Autodesk Inventor part; units mm, degrees
ref_plane "YZ Plane" through (0, 0, 0) normal (1, 0, 0) x (0, 1, 0)
ref_plane "XZ Plane" through (0, 0, 0) normal (0, 1, 0) x (-1, 0, 0)
ref_plane "XY Plane" through (0, 0, 0) normal (0, 0, 1) x (1, 0, 0)
sketch "Sketch1" plane through (0, 0, 0) normal (0, 0, 1) x (1, 0, 0)
  line L0 (0, 10) -> (0, 50)
  line L1 (0, 50) -> (60, 50)
  line L2 (60, 50) -> (60, 10)
  line L3 (60, 10) -> (40, 10)
  line L4 (40, 10) -> (40, 0)
  line L5 (40, 0) -> (20, 0)
  line L6 (20, 0) -> (20, 10)
  line L7 (20, 10) -> (0, 10)
  point P0 (0, 0)
  dimension "d0" = 40
  dimension "d1" = 60
  dimension "d2" = 20
  dimension "d3" = 20
extrude "Extrusion1" add sketch "Sketch1" along normal blind 35
sketch "Sketch2" plane through (0, 0, 35) normal (0, 0, 1) x (1, 0, 0)
  circle A0 centre (30, 5) radius 3
  line L0 (20, 10) -> (20, 0)
  line L1 (20, 0) -> (40, 0)
  point P0 (0, 0)
  point P1 (20, 5)
  point P2 (30, 0)
  dimension "d6" = 6
  dimension "d7" = 10
  dimension "d8" = 5
extrude "Extrusion2" cut sketch "Sketch2" against normal blind 35
properties part number "haraketli_cene"
Here's how the part is built. I have some questions about the finished solid (model axes, mm). A direction names the side the tool comes from. Coordinates: 2 decimals unless noted, no trailing zeros. Order: outer loops, then holes, each group sorted by start corner. A loop starts at its lowest first (then second) coordinate and runs counter-clockwise, first axis right, second up.
Item 1: If we section it at A-A, the plane x = 30: List the corners of the cut face in (y, z) for me, then the cut area to 3 significant figures.
Response values:
outline: (0, 0) - (2, 0) - (2, 35) - (0, 35) - close; (8, 0) - (50, 0) - (50, 35) - (8, 35) - close
area: 1,540 mm2
Item 2: I need wall thicknesses on probe 1 along Y at (x, z) = (30, 20); probe 2 along Y at (x, z) = (55.5, 5); probe 3 along X at (y, z) = (8.5, 1). Which ranges of each line are inside material? Lowest first, please.
Response values:
probe 1: y = 0 to 2, 8 to 50
probe 2: y = 10 to 50
probe 3: x = 20 to 40
Item 3: If we section it at B-B, the plane y = 5: List the corners of the cut face in (x, z) for me, then the cut area to 3 significant figures.
Response values:
outline: (20, 0) - (27, 0) - (27, 35) - (20, 35) - close; (33, 0) - (40, 0) - (40, 35) - (33, 35) - close
area: 490 mm2
Item 4: If we section it at C-C, the plane z = 27: List the corners of the cut face in (x, y) for me, then the cut area to 3 significant figures.
Response values:
outline: (0, 10) - (20, 10) - (20, 0) - (40, 0) - (40, 10) - (60, 10) - (60, 50) - (0, 50) - close; hole circle Ø6 at (30, 5)
area: 2,570 mm2
Item 5: Which directions (+Z, -Z, +X, -X, +Y, -Y) give clear straight access to the entire face, cutting with the end or side of a thin tool? Please do faces 1 (the face through (40, 5, 17)), 2 (the face through (20, 5, 17)), 3 (the face through (30, 31, 0)).
Response values:
face 1: +Z, -Z, +X, -Y
face 2: +Z, -Z, -X, -Y
face 3: -Z, +X, -X, +Y, -Y
Item 6: If we section it at D-D, the plane x = 46.5: List the corners of the cut face in (y, z) for me, then the cut area to 3 significant figures.
Response values:
outline: (10, 0) - (50, 0) - (50, 35) - (10, 35) - close
area: 1,400 mm2
Item 7: I'm going to push flat-ended pins straight in: pin 1 Ø2 at (x, y) = (49.5, 28) entering from -Z; pin 2 Ø6 at (y, z) = (6.5, 23) entering from -X; pin 3 Ø16 at (x, z) = (5.5, 19) entering from -Y; pin 4 Ø8 at (y, z) = (4, 19) entering from +X. Where does each tip first touch, or does it pass through?
Response values:
pin 1: stops at z = 0
pin 2: stops at x = 20
pin 3: stops at y = 10
pin 4: stops at x = 40
Item 8: Thinking about a two-plate mould opening in X: for faces 4 (the face through (30, 0, 17)), 5 (the face through (27, 5, 18)), 6 (the face through (0, 30, 17)), 7 (the face through (60, 30, 17)), which applies, pulls with the +X half, pulls with the -X half, needs draft (parallel to the pull), parting line crosses it, or undercut?
Response values:
face 4: needs draft
face 5: undercut
face 6: pulls with the -X half
face 7: pulls with the +X half
